Could you check a few things on this model? Use its own coordinates, in mm. Round coordinates to 2 decimals unless told otherwise and drop trailing zeros. One line per item, written item: value. Start each with the question number.
Q1. I'm going to push a flat-ended pin straight in: pin 1 Ø1.8 at (y, z) = (2.2, -97.8) entering from +X (3 decimals). Where does the tip first touch, or does it pass through?
Q2. Please list where these lines run through material, in increasing order: line 1 along Z through (x, y) = (2.4, 2.2); line 2 along Y through (x, z) = (1.35, -2.2); line 3 along Z through (x, y) = (1, 3).
Q3. Thinking about a two-plate mould opening in Z: for faces 1 (the face through (1.48, 0.6, -99.43)), 2 (the face through (1, 0, -51)), 3 (the face through (1.6, 2.2, -98.9)), which applies, released by +Z, released by -Z, zero draft, split by the parting line, or undercut?
Autodesk Inventor part; units mm, degrees
ref_plane "YZ Plane" through (0, 0, 0) normal (1, 0, 0) x (0, 1, 0)
ref_plane "XZ Plane" through (0, 0, 0) normal (0, 1, 0) x (-1, 0, 0)
ref_plane "XY Plane" through (0, 0, 0) normal (0, 0, 1) x (1, 0, 0)
sketch "Sketch1" plane through (0, 0, 0) normal (1, 0, 0) x (0, 1, 0)
  line L0 (2, 0) -> (48, 0)
  line L1 (50, -2) -> (50, -98)
  line L2 (48, -100) -> (2, -100)
  line L3 (0, -98) -> (0, -2)
  arc A0 (50, -2) -> (48, 0) centre (48, -2) ccw
  arc A1 (0, -98) -> (2, -100) centre (2, -98) ccw
  arc A2 (48, -100) -> (50, -98) centre (48, -98) ccw
  arc A3 (2, 0) -> (0, -2) centre (2, -2) ccw
  circle A4 centre (47.8, -2.2) radius 1.1
  line L4 (50, -50) -> (19.7358, -50) construction
  line L5 (25, 0) -> (25, -33.4431) construction
  circle A5 centre (47.8, -97.8) radius 1.1
  circle A6 centre (2.2, -2.2) radius 1.1
  circle A7 centre (2.2, -97.8) radius 1.1
  point P0 (0, 0)
  point P1 (50, -100)
  point P2 (50, 0)
  point P3 (0, -100)
  point P4 (2, -2)
  point P5 (2, -98)
  dimension "d0" = 50
  dimension "d1" = 100
  dimension "d2" = 2
  dimension "d3" = 2.2
  dimension "d4" = 2.2
  dimension "d5" = 2.2
extrude "Extrusion1" add sketch "Sketch1" along normal blind 3 contours L0 A0 L1 A2 L2 A1 L3 A3 | A4 | A5 | A6 | A7
hole "Hole1" at (0, 47.8, -2.2) at (0, 2.2, -2.2) at (0, 47.8, -97.8) at (0, 2.2, -97.8) direction (1, 0, 0) diameter 2.2 depth 6.3 tip angle 118
chamfer "Chamfer1" distance 0.2 angle 45 4 edges at (0, 2.2, -98.9) (0, 47.8, -98.9) (0, 2.2, -3.3) (0, 47.8, -3.3)
properties part number "ściana tylna"
Report:
1. pin 1: passes through
2. line 1: z = -100 to -98.9, -96.7 to -3.3, -1.1 to 0
2. line 2: y = 0 to 1.1, 3.3 to 46.7, 48.9 to 50
2. line 3: z = -100 to -98.55, -97.05 to -2.95, -1.45 to 0
3. face 1: released by -Z
3. face 2: zero draft
3. face 3: undercut
